Autodesk Inventor part; units mm, degrees
ref_plane "YZ Plane" through (0, 0, 0) normal (1, 0, 0) x (0, 1, 0)
ref_plane "XZ Plane" through (0, 0, 0) normal (0, 1, 0) x (-1, 0, 0)
ref_plane "XY Plane" through (0, 0, 0) normal (0, 0, 1) x (1, 0, 0)
sketch "Sketch1" plane through (0, 0, 0) normal (0, 1, 0) x (-1, 0, 0)
  line L0 (7.75, 9.55) -> (-7.75, 9.55)
  line L1 (-7.75, 9.55) -> (-7.75, -9.55)
  line L2 (-7.75, -9.55) -> (7.75, -9.55)
  line L3 (7.75, -9.55) -> (7.75, 9.55)
  line L4 (7.75, 9.55) -> (-7.75, -9.55) construction
  line L5 (-7.75, 9.55) -> (7.75, -9.55) construction
  point P0 (0, 0)
  dimension "d0" = 15.5
  dimension "d1" = 19.1
extrude "Extrusion1" add sketch "Sketch1" along normal blind 15.3
sketch "Sketch2" plane through (0, 0, 0) normal (0, -1, 0) x (1, 0, 0)
  line L0 (7.75, 9.55) -> (7.75, -9.55)
  line L1 (-7.75, 9.55) -> (7.75, 9.55)
  line L2 (-7.75, -9.55) -> (-7.75, 9.55)
  line L3 (7.75, -9.55) -> (-7.75, -9.55)
  circle A0 centre (-6, 6.15) radius 0.3
  circle A1 centre (6, 6.15) radius 0.3
  circle A2 centre (0, 8.15) radius 0.3
  circle A3 centre (-6, -6.55) radius 0.3
  circle A4 centre (6, -6.55) radius 0.28
  point P0 (0, 0)
  dimension "d4" = 0.6
  dimension "d5" = 0.6
  dimension "d6" = 0.6
  dimension "d9" = 6
  dimension "d10" = 6
  dimension "d11" = 0.6
  dimension "d12" = 0.56
  dimension "d13" = 2
  dimension "d14" = 1.4
  dimension "d15" = 2
  dimension "d18" = 12.7
  dimension "d19" = 12.7
extrude "Extrusion2" add sketch "Sketch2" along normal blind 6 contours A0 | A1 | A2 | A3 | A4
properties part number "relay_sdr-03vdc-sl-c" material "ABS Plastic"
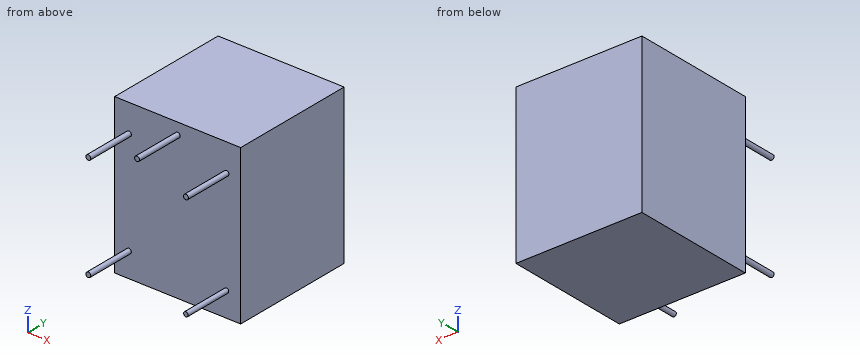
Build history of the part. All positions in model axes, mm. Round coordinates to 2 decimals unless told otherwise and drop trailing zeros. Write each loop counter-clockwise with the first axis right and the second up, starting at its lowest first coordinate (ties: lowest second). Pieces come first, ordered by that corner, then holes.
1) Band-saw the part on B-B, the plane z = 8.15. List the corners of the cut face in (x, y).
2) Band-saw the part on A-A, the plane y = -4.25. List the corners of the cut face in (x, z), and give its area (3 significant figures).
3) Band-saw the part on C-C, the plane x = 0. List the corners of the cut face in (y, z), and give its area (3 significant figures).
4) Pin check, flat tips, straight feed: pin 1 (4 mm diameter, centred on x = 5, z = -3.5, fed in from -Y); pin 2 (8 mm diameter, centred on y = -2, z = 0.5, fed in from +X). Stop position of each tip, or through.
5) Band-saw the part on D-D, the plane z = 6.15. List the corners of the cut face in (x, y).
6) Drill centre line: probe 1 along Y at (x, z) = (-6.25, 2.5). Where is it in solid material? Low to high.
Ans:
1. outline: (-7.75, 0) - (-0.3, 0) - (-0.3, -6) - (0.3, -6) - (0.3, 0) - (7.75, 0) - (7.75, 15.3) - (-7.75, 15.3) - close
2. outline: circle Ø0.6 at (-6, -6.55); circle Ø0.6 at (-6, 6.15); circle Ø0.6 at (0, 8.15); circle Ø0.6 at (6, 6.15); circle Ø0.56 at (6, -6.55)
2. area: 1.38 mm2
3. outline: (-6, 7.85) - (0, 7.85) - (0, -9.55) - (15.3, -9.55) - (15.3, 9.55) - (0, 9.55) - (0, 8.45) - (-6, 8.45) - close
3. area: 296 mm2
4. pin 1: stops at y = 0
4. pin 2: stops at x = 7.75
5. outline: (-7.75, 0) - (-6.3, 0) - (-6.3, -6) - (-5.7, -6) - (-5.7, 0) - (5.7, 0) - (5.7, -6) - (6.3, -6) - (6.3, 0) - (7.75, 0) - (7.75, 15.3) - (-7.75, 15.3) - close
6. probe 1: y = 0 to 15.3
